Geometry check sheet. Reference: the model listing, model coordinates, mm. A direction names the side the tool comes from. Give positions to 0.01 mm unless a question says otherwise; leave off trailing zeros. Loops run counter-clockwise (first coordinate to the right, second up) from the corner with the lowest first, then second, coordinate; pieces in that order, holes last. Notation, with made-up numbers: (61.25, 21) -> (99.25, 21) arc R14 ccw to (99.25, 38) -> close; hole circle Ø7 at (46.5, 36.5). An arc over 180 degrees is marked (long way). Write item = value, one per line. Start each with the question number.
```python
from build123d import *

# Parameters (mm, degrees)
BOSS_EXTRUDE1_DEPTH = 58.42
SKETCH3_W           = 99.999999898
SKETCH3_H           = 90.000000086
CUT_EXTRUDE1_DEPTH  = 55.245
SKETCH5_R           = 3.175
SKETCH5_R_2         = 1.5875
BOSS_EXTRUDE2_DEPTH = 22.86
BOSS_EXTRUDE3_DEPTH = 58.42
SKETCH8_R           = 2.38125
CUT_EXTRUDE2_DEPTH  = 12.7


with BuildPart() as part:
    # Sketch1 → Boss-Extrude1 (new body)
    with BuildSketch(Plane(origin=(0, 0, 0), x_dir=(1, 0, 0), z_dir=(0, 1, 0))):
        with BuildLine():
            Line((3.175, 0), (103.174999898, 0))
            ThreePointArc((103.174999898, 0), (105.420063928, 0.92993597), (106.349999898, 3.175))
            Line((106.349999898, 3.175), (106.349999898, 93.175000086))
            ThreePointArc((106.349999898, 93.175000086), (105.420063928, 95.420064116), (103.174999898, 96.350000086))
            Line((103.174999898, 96.350000086), (3.175, 96.350000086))
            ThreePointArc((3.175, 96.350000086), (0.92993597, 95.420064116), (0, 93.175000086))
            Line((0, 93.175000086), (0, 3.175))
            ThreePointArc((0, 3.175), (0.92993597, 0.92993597), (3.175, 0))
        make_face()
    extrude(amount=BOSS_EXTRUDE1_DEPTH)

    # Sketch3 → Cut-Extrude1 (cut)
    with BuildSketch(Plane(origin=(0, 58.42, 0), x_dir=(1, 0, 0), z_dir=(0, 1, 0))):
        with Locations((53.174999949, 48.175000043)):
            Rectangle(SKETCH3_W, SKETCH3_H)
    extrude(amount=-CUT_EXTRUDE1_DEPTH, mode=Mode.SUBTRACT)

    # Sketch5 → Boss-Extrude2 (add)
    # profile 1 of 2: a face of its own
    with BuildSketch(Plane(origin=(0, 3.175, 0), x_dir=(1, 0, 0), z_dir=(0, 1, 0))):
        with Locations(Location((66.303499949, 10.055000043, 0), (0, 0, 270))):
            Circle(SKETCH5_R)
        with Locations(Location((66.303499949, 10.055000043, 0), (0, 0, 270))):
            Circle(SKETCH5_R_2, mode=Mode.SUBTRACT)
    # profile 2 of 2: a face of its own
    with BuildSketch(Plane(origin=(0, 3.175, 0), x_dir=(1, 0, 0), z_dir=(0, 1, 0))):
        with Locations(Location((9.890999949, 86.717500043, 0), (0, 0, 270))):
            Circle(SKETCH5_R)
        with Locations(Location((9.890999949, 86.717500043, 0), (0, 0, 270))):
            Circle(SKETCH5_R_2, mode=Mode.SUBTRACT)
    extrude(amount=BOSS_EXTRUDE2_DEPTH)

    # Sketch7 → Boss-Extrude3 (add)
    with BuildSketch(Plane.XZ):
        with BuildLine():
            Line((3.175, -102.700000086), (103.174999898, -102.700000086))
            ThreePointArc((103.174999898, -102.700000086), (109.910191989, -99.910192177), (112.699999898, -93.175000086))
            Line((112.699999898, -93.175000086), (112.699999898, -3.175))
            ThreePointArc((112.699999898, -3.175), (109.910191989, 3.560192091), (103.174999898, 6.35))
            Line((103.174999898, 6.35), (3.175, 6.35))
            ThreePointArc((3.175, 6.35), (-3.560192091, 3.560192091), (-6.35, -3.175))
            Line((-6.35, -3.175), (-6.35, -93.175000086))
            ThreePointArc((-6.35, -93.175000086), (-3.560192091, -99.910192177), (3.175, -102.700000086))
        make_face()
        with BuildLine():
            Line((3.175, -96.350000086), (103.174999898, -96.350000086))
            ThreePointArc((103.174999898, -96.350000086), (105.420063928, -95.420064116), (106.349999898, -93.175000086))
            Line((106.349999898, -93.175000086), (106.349999898, -3.175))
            ThreePointArc((106.349999898, -3.175), (105.420063928, -0.92993597), (103.174999898, 0))
            Line((103.174999898, 0), (3.175, 0))
            ThreePointArc((3.175, 0), (0.92993597, -0.92993597), (0, -3.175))
            Line((0, -3.175), (0, -93.175000086))
            ThreePointArc((0, -93.175000086), (0.92993597, -95.420064116), (3.175, -96.350000086))
        make_face(mode=Mode.SUBTRACT)
    extrude(amount=-BOSS_EXTRUDE3_DEPTH)

    # Sketch8 → Cut-Extrude2 (cut)
    with BuildSketch(Plane(origin=(0, 58.42, 0), x_dir=(1, 0, 0), z_dir=(0, 1, 0))):
        with Locations(Location((-1.5875, 48.175000043, 0), (0, 0, 270))):
            Circle(SKETCH8_R)
        with Locations(Location((53.174999949, 97.937500086, 0), (0, 0, 270))):
            Circle(SKETCH8_R)
        with Locations(Location((107.937499898, 48.175000043, 0), (0, 0, 90))):
            Circle(SKETCH8_R)
        with Locations(Location((53.174999949, -1.5875, 0), (0, 0, 90))):
            Circle(SKETCH8_R)
    extrude(amount=-CUT_EXTRUDE2_DEPTH, mode=Mode.SUBTRACT)


solid = part.part
```
1) Draft check along X on faces 3 (the flat face through (-6.35, 29, -48)), 4 (the flat face through (103.175, 31, -48)), 5 (the cylindrical face through (109.84, 28.8, -99.98)). Enter one of: released by +X, released by -X, zero draft, split by the parting line, or undercut.
2) Section check D-D (x = 42). Enter the section's corners in (y, z) (3 decimals).
3) Section check B-B (z = -76). Enter the section's corners in (x, y) (3 decimals), plus the area to 3 significant figures.
4) Tool access check on faces 1 (the flat face through (9, 26.035, -85)), 2 (the flat face through (54, 29, 6.35)). Record the directions out of +Z, -Z, +X, -X, +Y, -Y that give a thin tool (end or side, any length) a straight path to the whole face; none if there is none.
5) Thickness scan on line 1 (X direction, y = 31.5, z = -55) (3 decimals); line 2 (Z direction, x = 46.5, y = 53) (3 decimals); line 3 (Z direction, x = 12.5, y = 17) (3 decimals). Record the ranges inside material, lowest first.
6) Section check C-C (y = 29). Enter the section's corners in (x, z) (3 decimals).
7) Depth check by flat-ended pin: pin 1 Ø1.9 at (x, z) = (9.89, -86.72) entering from +Y (3 decimals); pin 2 Ø1.9 at (x, z) = (66, -11) entering from +Y (3 decimals); pin 3 Ø1.4 at (x, z) = (108, -48) entering from +Y. Enter the tip coordinate at first touch or a pass-through.
8) Section check A-A (y = 17). Give the number of separate pieces and of enclosed holes in the cut face, plus the area to 3 significant figures.
Check result:
q1.face_3 = released by -X
q1.face_4 = undercut
q1.face_5 = released by +X
q2.outline = (0, -102.7) -> (58.42, -102.7) -> (58.42, -93.175) -> (3.175, -93.175) -> (3.175, -3.175) -> (58.42, -3.175) -> (58.42, 6.35) -> (0, 6.35) -> close
q3.outline = (-6.35, 0) -> (112.7, 0) -> (112.7, 58.42) -> (103.175, 58.42) -> (103.175, 3.175) -> (3.175, 3.175) -> (3.175, 58.42) -> (-6.35, 58.42) -> close
q3.area = 1,430 mm2
q4.face_1 = +Y
q4.face_2 = +Z, +X, -X, +Y, -Y
q5.line_1 = -6.35 to 3.175, 103.175 to 112.7
q5.line_2 = -102.7 to -93.175, -3.175 to 6.35
q5.line_3 = -102.7 to -93.175, -88.527 to -84.908, -3.175 to 6.35
q6.outline = (-6.35, -93.175) arc R9.525 ccw to (3.175, -102.7) -> (103.175, -102.7) arc R9.525 ccw to (112.7, -93.175) -> (112.7, -3.175) arc R9.525 ccw to (103.175, 6.35) -> (3.175, 6.35) arc R9.525 ccw to (-6.35, -3.175) -> close; hole (3.175, -93.175) -> (103.175, -93.175) -> (103.175, -3.175) -> (3.175, -3.175) -> close
q7.pin_1 = 3.175
q7.pin_2 = 26.035
q7.pin_3 = 45.72
q8.separate_pieces = 3
q8.enclosed_holes = 3
q8.area = 3,950 mm2
